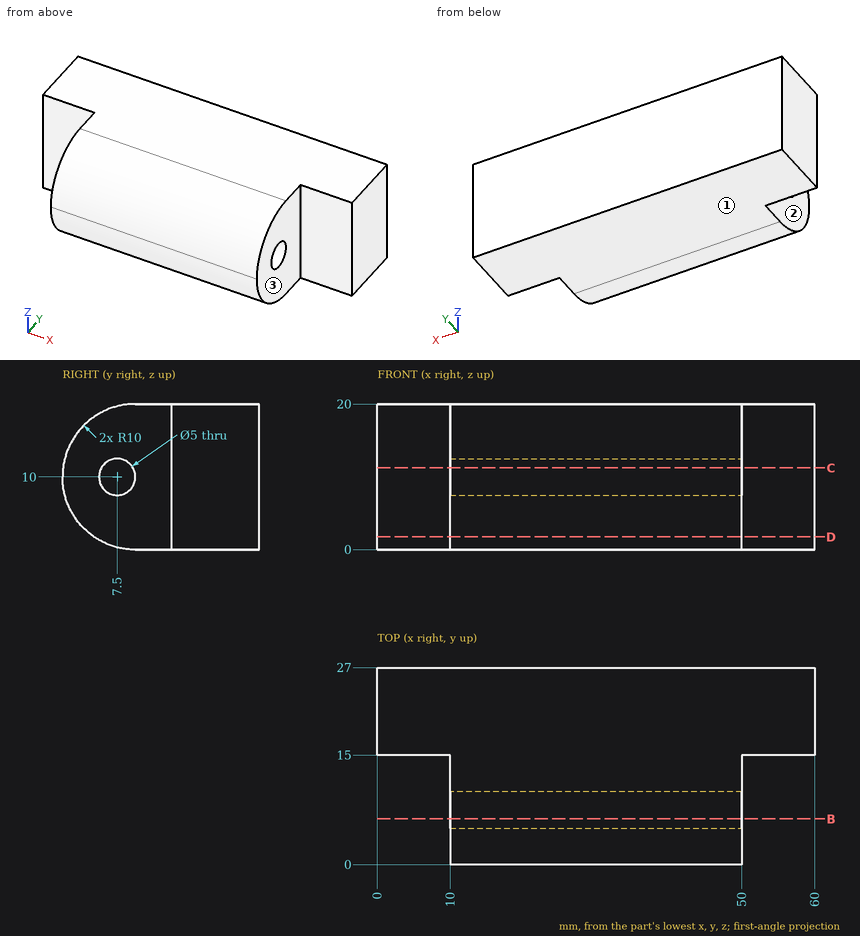
Part print with two shaded views. Sizes in mm from the minimum x, y, z corner. A direction names the side the tool comes from. Round coordinates to 2 decimals unless told otherwise and drop trailing zeros. Loops run counter-clockwise (first coordinate to the right, second up) from the corner with the lowest first, then second, coordinate; pieces in that order, holes last. Notation, with made-up numbers: M 37.5,51.25 L 91.5,51.25 A22 cw 91.5,89.25 Z; hole C -1,-26.5 d9. An arc over 180 degrees is marked long. Put each result on its own line as item: value. Start each with the question number.
Item 1: Drill centre lines: line 1 along X through (y, z) = (10.25, 15); line 2 along Z through (x, y) = (31.5, 7.5); line 3 along Y through (x, z) = (40.5, 11.25) (1 decimal). Where is each one in solid material? Low to high.
Item 2: Cut at B-B (y = 6.25). List the corners of the cut face in (x, z) (3 decimals).
Item 3: Cut at D-D (z = 1.75). List the corners of the cut face in (x, y), then the cut area to 3 significant figures.
Item 4: 3-axis set-ups, long thin cutter, end or side, ignore diameter. For the marked faces 1, 2 and 3: which of +Z, -Z, +X, -X, +Y, -Y reach the whole face in a straight line?
Item 5: Cut at C-C (z = 11.25). List the corners of the cut face in (x, y) (1 decimal).
Item 6: Drop flat-ended pins along their axis: P1, Ø11, axis at x = 56, z = 7, coming from the -Y side; P2, Ø12, axis at y = 7, z = 10, coming from the +X side; P3, Ø1, axis at x = 37.5, y = 3, coming from the +Z side; P4, Ø3, axis at y = 7.5, z = 10, coming from the -X side. Give the stop position or say it passes through.
Answer block:
1. line 1: 10 to 50
1. line 2: 0.32 to 7.5, 12.5 to 19.68
1. line 3: 0.1 to 5.3, 9.7 to 27
2. outline: M 10,0.73 L 50,0.73 L 50,7.835 L 10,7.835 Z; M 10,12.165 L 50,12.165 L 50,19.27 L 10,19.27 Z
3. outline: M 0,15 L 10,15 L 10,4.35 L 50,4.35 L 50,15 L 60,15 L 60,27 L 0,27 Z
3. area: 1,150 mm2
4. face 1: -Z, +X, -X, +Y, -Y
4. face 2: +Z, -Z, -X, -Y
4. face 3: +Z, -Z, +X, -Y
5. outline: M 0,15 L 10,15 L 10,9.7 L 50,9.7 L 50,15 L 60,15 L 60,27 L 0,27 Z; M 10,0.1 L 50,0.1 L 50,5.3 L 10,5.3 Z
6. P1: y = 15
6. P2: x = 50
6. P3: z = 17.6
6. P4: through
